```python
from build123d import *

# Parameters (mm, degrees)
BOX_W                     = 0.6
BOX_H                     = 0.4
BOX_DEPTH                 = 2.5
BOX002_W                  = 0.6
BOX002_H                  = 0.4
BOX002_DEPTH              = 2.5
CYLINDER002_R             = 5.5
CYLINDER002_DEPTH         = 2
FUSION002_PLACEMENT_ANGLE = 90
BOX001_W                  = 6
BOX001_H                  = 15
BOX001_DEPTH              = 0.5
CUT005_PLACEMENT_ANGLE    = 90
PAD003_DEPTH              = 5
SKETCH004_R               = 1.5
SKETCH004_R_2             = 1.365842
PAD004_DEPTH              = 5
FILLET_R                  = 0.3
FUSION001_PLACEMENT_ANGLE = 90


with BuildPart() as obj1:
    # Box → Box (new body)
    with BuildSketch(Plane(origin=(2.95, -0.2, -2), x_dir=(1, 0, 0), z_dir=(0, 0, 1))):
        with Locations((0.3, 0.2)):
            Rectangle(BOX_W, BOX_H)
    extrude(amount=BOX_DEPTH)


with BuildPart() as obj2:
    # Box002 → Box002 (new body)
    with BuildSketch(Plane(origin=(-3.55, -0.2, -2), x_dir=(1, 0, 0), z_dir=(0, 0, 1))):
        with Locations((0.3, 0.2)):
            Rectangle(BOX002_W, BOX002_H)
    extrude(amount=BOX002_DEPTH)


with BuildPart() as interior_buzzer:
    # Cylinder002 → Cylinder002 (new body)
    with BuildSketch(Plane.XY):
        Circle(CYLINDER002_R)
    extrude(amount=CYLINDER002_DEPTH)

    # Fusion002: union obj1, obj2
    add(obj1.part)
    add(obj2.part)


with BuildPart() as interior_buzzer_1:
    # Fusion002 placement: moved
    add(interior_buzzer.part.moved(Location((0, 0, 0.5))).rotate(Axis((0, 0, 0.5), (0, 0, 1)), FUSION002_PLACEMENT_ANGLE))


with BuildPart() as obj3:
    # Box001 → Box001 (new body)
    with BuildSketch(Plane(origin=(-3, -7, 0), x_dir=(1, 0, 0), z_dir=(0, 0, 1))):
        with Locations((3, 7.5)):
            Rectangle(BOX001_W, BOX001_H)
    extrude(amount=BOX001_DEPTH)


with BuildPart() as obj4:
    # Sketch002 → Revolution001 (revolve)
    with BuildSketch(Plane.XZ):
        Polygon((5.5, 2.5), (5.5, 0), (6, 0), (6, 2), (5.75, 2), (5.75, 2.5), align=None)
    revolve(axis=Axis((0, 0, 0), (0, 0, 1)))

    # Cut005: cut obj3
    add(obj3.part, mode=Mode.SUBTRACT)


with BuildPart() as obj4_1:
    # Cut005 placement: moved
    add(obj4.part.rotate(Axis((0, 0, 0), (0, 0, 1)), CUT005_PLACEMENT_ANGLE))


with BuildPart() as obj5:
    # Sketch005 → Pad003 (new body)
    with BuildSketch(Plane.XY.offset(9.5)):
        Polygon((-0.15, 5.014959), (0.15, 5.014959), (0.15, 4.051414), (1.113545, 4.051414), (1.113545, 3.751414), (0.15, 3.751414), (0.15, 2.787869), (-0.15, 2.787869), (-0.15, 3.751414), (-1.113545, 3.751414), (-1.113545, 4.051414), (-0.15, 4.051414), align=None)
    extrude(amount=PAD003_DEPTH)


with BuildPart() as obj6:
    # Sketch004 → Pad004 (new body)
    with BuildSketch(Plane.XY.offset(9.5)):
        with Locations((0, 3.923361)):
            Circle(SKETCH004_R)
        with Locations((0, 3.923361)):
            Circle(SKETCH004_R_2, mode=Mode.SUBTRACT)
    extrude(amount=PAD004_DEPTH)


with BuildPart() as buzzer:
    # Sketch003 → Revolution (revolve)
    with BuildSketch(Plane.XZ):
        Polygon((1.3, 9.57124), (6, 9.57124), (6, 2.17124), (5.75, 2.17124), (5.75, 2.57124), (5.5, 2.57124), (5.5, 9.07124), (1.3, 9.07124), align=None)
    revolve(axis=Axis((0, 0, 0), (0, 0, 1)))

    # Fillet
    fillet_edges = [buzzer.edges().sort_by_distance(p)[0] for p in [
        (-6, 0, 9.57124),
    ]]
    fillet(fillet_edges, radius=FILLET_R)

    # Cut004: cut obj6
    add(obj6.part, mode=Mode.SUBTRACT)

    # Cut003: cut obj5
    add(obj5.part, mode=Mode.SUBTRACT)

    # Fusion001: union Interior_buzzer, obj4
    add(interior_buzzer_1.part)
    add(obj4_1.part)


with BuildPart() as buzzer_1:
    # Fusion001 placement: moved
    add(buzzer.part.moved(Location((0, 4, 1.7))).rotate(Axis((0, 4, 1.7), (0, 0, 1)), FUSION001_PLACEMENT_ANGLE))


solid = buzzer_1.part
```
Can you work these out from the model? Positions are in its coordinate system, mm. A direction names the side the tool comes from. Coordinates: 2 decimals unless noted, no trailing zeros. Loops run counter-clockwise (first coordinate to the right, second up) from the corner with the lowest first, then second, coordinate; pieces in that order, holes last.
Item 1: If we mould it in two halves opening along Y, with no side actions, what happens to faces 1 (the face through (5.5, 3.9, 1.9)), 2 (the face through (0.78, -1.95, 2.71)), 3 (the face through (1.2, 2.8, 11.271))? For each: released by +Y, released by -Y, zero draft, split by the parting line, or undercut.
Answers below:
face 1: undercut
face 2: split by the parting line
face 3: zero draft
Item 2: Which directions (+Z, -Z, +X, -X, +Y, -Y) give clear straight access to the entire face, cutting with the end or side of a thin tool? Please do faces 4 (the face through (-5.5, 4.1, 1.9)), 5 (the face through (2.11, 9.08, 7.57)), 6 (the face through (2.3, 9.54, 7.37)), 7 (the face through (-0.39, 5.24, 11.02)).
Answers below:
face 4: -Z
face 5: none
face 6: +Z, -Z
face 7: +Z
Item 3: Suppose I cut it at B-B (x = 0). Please give me the cut outline in (y, z), then the cut area to 3 significant figures.
Answers below:
outline: (-2, 2.2) - (10, 2.2) - (10, 3.7) - (9.75, 3.7) - (9.75, 3.87) - (10, 3.87) - (10, 10.97) arc R0.3 ccw to (9.7, 11.27) - (5.3, 11.27) - (5.3, 10.77) - (9.5, 10.77) - (9.5, 4.27) - (9.75, 4.27) - (9.75, 4.2) - (-1.75, 4.2) - (-1.75, 4.27) - (-1.5, 4.27) - (-1.5, 10.77) - (2.7, 10.77) - (2.7, 11.27) - (-1.7, 11.27) arc R0.3 ccw to (-2, 10.97) - (-2, 3.87) - (-1.75, 3.87) - (-1.75, 3.7) - (-2, 3.7) - close
area: 35.1 mm2
Item 4: Suppose I cut it at A-A (z = 5.5). Please give me the cut outline in (x, y), then the cut area to 3 significant figures.
Answers below:
outline: circle Ø12 at (0, 4); hole circle Ø11 at (0, 4)
area: 18.1 mm2
Item 5: Please list where these lines run through material, in increasing order: L1, parallel to Z at x = 1.25, y = 0.5; L2, parallel to X at y = 4, z = 10.95; L3, parallel to X at y = 1.75, z = 7.5.
Answers below:
L1: z = 2.2 to 4.2, 10.77 to 11.27
L2: x = -6 to -1.3, 1.3 to 6
L3: x = -5.56 to -5.02, 5.02 to 5.56
Item 6: I'm going to push flat-ended pins straight in: pin 1 (3.5 mm diameter, centred on x = -3.92, y = 4, fed in from -Z); pin 2 (1 mm diameter, centred on x = 3, z = 3, fed in from +Y); pin 3 (0.7 mm diameter, centred on x = -3.5, z = 1.5, fed in from -Y); pin 4 (1.5 mm diameter, centred on x = 4.5, y = 6.5, fed in from -Z). Where does each tip first touch, or does it pass through?
Answers below:
pin 1: stops at z = 0.2
pin 2: stops at y = 9.45
pin 3: stops at y = -1.07
pin 4: stops at z = 1.7
Item 7: Suppose I cut it at C-C (z = 3). Please give me the cut outline in (x, y), then the cut area to 3 significant figures.
Answers below:
outline: circle Ø12 at (0, 4)
area: 113 mm2
